```python
from build123d import *

# Parameters (mm, degrees)
SKETCH1_R  = 6.5
BASE_DEPTH = 2.54


with BuildPart() as part:
    # Sketch1 → Base (new body)
    with BuildSketch(Plane(origin=(0, 0, 0), x_dir=(0, 0, -1), z_dir=(1, 0, 0))):
        with BuildLine():
            Line((9, -4), (9, 8))
            Line((9, 8), (-9, 8))
            Line((-9, 8), (-9, -4))
            Line((-9, -4), (-6.945502142, -4))
            Line((-6.945502142, -4), (-6.945502142, -6.54))
            ThreePointArc((-6.945502142, -6.54), (0, -9.54), (6.945502142, -6.54))
            Line((6.945502142, -6.54), (6.945502142, -4))
            Line((6.945502142, -4), (9, -4))
        make_face()
        Circle(SKETCH1_R, mode=Mode.SUBTRACT)
    extrude(amount=BASE_DEPTH)


solid = part.part
```
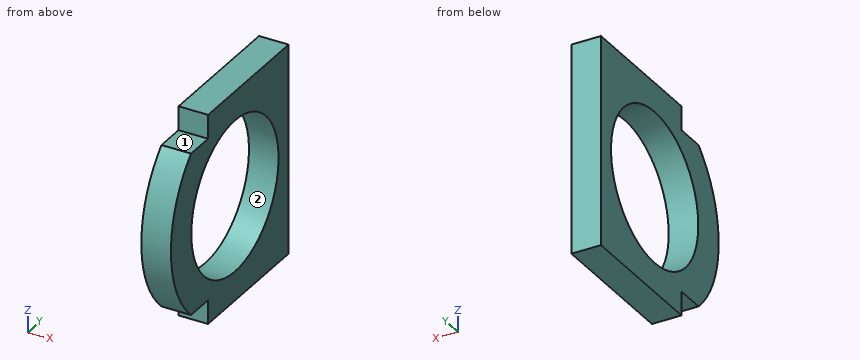
For this review, take the finished solid that the model builds, in its own axes (mm). Face numbers are marked on the shaded views. A direction names the side the tool comes from. Give positions to 0.01 mm unless a question says otherwise; leave off trailing zeros. Loops run counter-clockwise (first coordinate to the right, second up) from the corner with the lowest first, then second, coordinate; pieces in that order, holes last. Notation, with made-up numbers: M 21,87 L 32,87 A20 ccw 32,96 Z; hole C -28.5,-6 d5. An arc over 180 degrees is marked long. One line per item, written item: value. Start each with the question number.
Q1. Machinability: for the marked faces 1 and 2, which of the approach directions +Z, -Z, +X, -X, +Y, -Y give a long, thin tool a straight path to every point of the face, cutting with its end or side? Answer none if there is none.
Q2. For L1, parallel to Y at x = 1.25, z = 0; L2, parallel to Z at x = 1.8, y = -3; L3, parallel to Z at x = 2.2, y = 2.25, list the stretches that pass through material, from the lowest coordinate up.
Q3. Clearance check with flat-ended pins moving along their axes: pin 1 Ø1.5 at (x, z) = (1.5, -3) entering from -Y; pin 2 Ø8 at (y, z) = (5.5, -2) entering from -X; pin 3 Ø1.3 at (x, y) = (1, -5) entering from -Z; pin 4 Ø0.6 at (x, z) = (1.5, -8.5) entering from -Y. State where each tip first meets the part, or that it passes through.
Q4. Add section C-C (x = 1.05). Give the boundary of the cut face in (y, z).
Q5. Add section A-A (y = 0). Give the boundary of the cut face in (x, z), and give its area (3 significant figures).
Q6. Add section B-B (z = 0). Give the boundary of the cut face in (x, y).
Reply:
1. face 1: +Z, +X, -X, -Y
1. face 2: +X, -X
2. L1: -9.54 to -6.5, 6.5 to 8
2. L2: -9 to -5.77, 5.77 to 9
2. L3: -9 to -6.1, 6.1 to 9
3. pin 1: y = -9.27
3. pin 2: x = 0
3. pin 3: z = -6.95
3. pin 4: y = -4
4. outline: M -6.54,-6.95 L -4,-6.95 L -4,-9 L 8,-9 L 8,9 L -4,9 L -4,6.95 L -6.54,6.95 A9.54 ccw Z; hole C 0,0 d13
5. outline: M 0,-9 L 2.54,-9 L 2.54,-6.5 L 0,-6.5 Z; M 0,6.5 L 2.54,6.5 L 2.54,9 L 0,9 Z
5. area: 12.7 mm²
6. outline: M 0,-9.54 L 2.54,-9.54 L 2.54,-6.5 L 0,-6.5 Z; M 0,6.5 L 2.54,6.5 L 2.54,8 L 0,8 Z
